```python
from build123d import *

# Parameters (mm, degrees)
SKETCH1_R               = 3
BOSS_EXTRUDE1_DEPTH     = 7
BOSS_EXTRUDE2_START     = -12
SKETCH2_R               = 3
BOSS_EXTRUDE2_DEPTH     = 12
SKETCH2_4_R             = 6
SKETCH2_4_R_2           = 3
BOSS_EXTRUDE3_DEPTH     = 10
CUT_EXTRUDE1_DEPTH      = 41.816663264
CUT_EXTRUDE1_DEPTH_BACK = 41.816663264
SKETCH4_R               = 1.5
SKETCH6_R               = 1.5
CUT_EXTRUDE2_DEPTH      = 44.485629849


with BuildPart() as part:
    # Sketch1 → Boss-Extrude1 (new body)
    with BuildSketch(Plane.YZ):
        with BuildLine():
            Line((-5.969924623, 30.6), (-8.954886934, 0.9))
            ThreePointArc((-8.954886934, 0.9), (0, -9), (8.954886934, 0.9))
            Line((8.954886934, 0.9), (5.969924623, 30.6))
            ThreePointArc((5.969924623, 30.6), (0, 36), (-5.969924623, 30.6))
        make_face()
        with Locations(Location((0, 0, 0), (0, 0, 270))):
            Circle(SKETCH1_R, mode=Mode.SUBTRACT)
        with Locations(Location((0, 30, 0), (0, 0, 270))):
            Circle(SKETCH1_R, mode=Mode.SUBTRACT)
    extrude(amount=BOSS_EXTRUDE1_DEPTH)

    # Sketch2 → Boss-Extrude2 (add)
    with BuildSketch(Plane.YZ.offset(7).offset(BOSS_EXTRUDE2_START)):
        with BuildLine():
            ThreePointArc((-5.969924623, 30.6), (-0.30037665, 24.007523561), (6, 30))
            ThreePointArc((6, 30), (5.992476439, 30.30037665), (5.969924623, 30.6))
            ThreePointArc((5.969924623, 30.6), (0, 36), (-5.969924623, 30.6))
        make_face()
        with Locations(Location((0, 30, 0), (0, 0, 270))):
            Circle(SKETCH2_R, mode=Mode.SUBTRACT)
    extrude(amount=BOSS_EXTRUDE2_DEPTH)

    # Sketch2_4 → Boss-Extrude3 (add)
    with BuildSketch(Plane.YZ.offset(7)):
        with Locations(Location((0, 0, 0), (0, 0, 270))):
            Circle(SKETCH2_4_R)
        with Locations(Location((0, 0, 0), (0, 0, 270))):
            Circle(SKETCH2_4_R_2, mode=Mode.SUBTRACT)
    extrude(amount=BOSS_EXTRUDE3_DEPTH)

    # Sketch4 → Cut-Extrude1 (cut, two sides: drawn at the far end of the back side and taken through both)
    with BuildSketch(Plane(origin=(0, 0, 0), x_dir=(-1, 0, 0), z_dir=(0, 1, 0)).offset(-CUT_EXTRUDE1_DEPTH_BACK)):
        with Locations(Location((-12, 0, 0), (0, 0, 90))):
            Circle(SKETCH4_R)
    extrude(amount=CUT_EXTRUDE1_DEPTH + CUT_EXTRUDE1_DEPTH_BACK, mode=Mode.SUBTRACT)

    # Sketch6 → Cut-Extrude2 (cut, through all)
    with BuildSketch(Plane(origin=(0, 0, 30), x_dir=(0, 1, 0), z_dir=(0, 0, 1))):
        with Locations(Location((0, 0, 0), (0, 0, 90))):
            Circle(SKETCH6_R)
    extrude(amount=CUT_EXTRUDE2_DEPTH, mode=Mode.SUBTRACT)


solid = part.part
```
Could you check a few things on this model? Use its own coordinates, in mm. A direction names the side the tool comes from. Coordinates: 2 decimals unless noted, no trailing zeros. Write each loop counter-clockwise with the first axis right and the second up, starting at its lowest first coordinate (ties: lowest second). Pieces come first, ordered by that corner, then holes. Notation, with made-up numbers: M -27,20 L 3,20 A17 cw 3,51 Z; hole C -35,48.5 d10. An arc over 180 degrees is marked long. Answer as CSV lines item,"result". Start each with the question number.
1) Please list where these lines run through material, in increasing order: line 1 (Z direction, x = 5, y = -2); line 2 (X direction, y = -4.6, z = 0); line 3 (Z direction, x = 7.5, y = 0.25). Write a range as from..to.
2) For P1, Ø2, axis at x = 11.5, z = -2, coming from the +Y side; P2, Ø2.5, axis at x = 0, y = 0, coming from the +Z side; P3, Ø5, axis at x = 6.5, y = -4, coming from the +Z side; P4, Ø3.5, axis at y = 0, z = 30, coming from the -X side, each with a flat end and sliding along its axis, tell me the tip position at first contact or that it passes through.
3) We'd pull the mould along Z, two halves only. Please class faces 3 (the flat face through (3.451, 7.483, 15.542)), 4 (the cylindrical face through (11.93, -5.323, -2.769)), 5 (the cylindrical face through (12.07, -4.33, -1.5)): +Z half, -Z half, draft (parallel to the pull), parting line (faces both ways), or undercut.
4) I want a section at B-B, the plane x = 12. Please give me the cut outline in (y, z), and give its area (3 significant figures).
5) I want a section at A-A, the plane y = 0. Please give me the cut outline in (x, z), and give its area (3 significant figures).
6) For faces 1 (the cylindrical face through (-1.43, -0.45, 34.28)), 2 (the flat face through (-5, 1, 33)), which set-ups out of +Z, -Z, +X, -X, +Y, -Y let a thin tool reach every point of the face, with its end or its side?
7) I want a section at D-D, the plane x = 5.75. Please give me the cut outline in (y, z).
8) I want a section at C-C, the plane z = 29. Please give me the cut outline in (x, y).
Data:
1,line 1,"z = -8.77..-2.24, 2.24..27.76, 32.24..35.66"
1,line 2,"x = 0..10.5, 13.5..17"
1,line 3,"z = -5.99..-2.99, 2.99..5.99"
2,P1,"stops at y = 5.89"
2,P2,"stops at z = 27.27"
2,P3,"stops at z = 35.81"
2,P4,"passes through"
3,face 3,"+Z half"
3,face 4,"parting line"
3,face 5,"undercut"
4,outline,"M -5.81,-1.5 A6 ccw 5.81,-1.5 L 2.6,-1.5 A3 cw -2.6,-1.5 Z; M -5.81,1.5 L -2.6,1.5 A3 cw 2.6,1.5 L 5.81,1.5 A6 ccw Z"
4,area,"66.4 mm^2"
5,outline,"M -5,24 L 0,24 L 0,3 L 17,3 L 17,6 L 7,6 L 7,27 L -5,27 Z; M -5,33 L -1.5,33 L -1.5,36 L -5,36 Z; M 0,-9 L 7,-9 L 7,-6 L 17,-6 L 17,-3 L 0,-3 Z; M 1.5,33 L 7,33 L 7,36 L 1.5,36 Z"
5,area,"312 mm^2"
6,face 1,"+Z"
6,face 2,"+Z, -Z, -X, +Y, -Y"
7,outline,"M -8.95,0.9 A9 ccw long 8.95,0.9 L 5.97,30.6 A6 ccw -5.97,30.6 Z; hole C 0,0 d6; hole C 0,30 d6"
8,outline,"M -5,-5.92 L 0,-5.92 L 0,-6.13 L 7,-6.13 L 7,-2.83 L -5,-2.83 Z; M -5,2.83 L 7,2.83 L 7,6.13 L 0,6.13 L 0,5.92 L -5,5.92 Z"
